from build123d import *

# Parameters (mm, degrees)
BOSS_EXTRUDE1_DEPTH = 0.75
SKETCH2_R           = 15.265
CUT_EXTRUDE1_DEPTH  = 47.8


with BuildPart() as part:
    # Sketch1 → Boss-Extrude1 (new body, symmetric)
    with BuildSketch(Plane.XY):
        Polygon((0, 15.245), (12, 41.045), (-34.1, 41.045), (-46.8, 15.245), align=None)
    extrude(amount=BOSS_EXTRUDE1_DEPTH, both=True)

    # Sketch2 → Cut-Extrude1 (cut, through all)
    with BuildSketch(Plane(origin=(0, 0, 0), x_dir=(0, 0, -1), z_dir=(1, 0, 0))):
        Circle(SKETCH2_R)
    extrude(amount=-CUT_EXTRUDE1_DEPTH, mode=Mode.SUBTRACT)


solid = part.part
Could you check a few things on this model? Use its own coordinates, in mm. Coordinates: 2 decimals unless noted, no trailing zeros. Loops run counter-clockwise (first coordinate to the right, second up) from the corner with the lowest first, then second, coordinate; pieces in that order, holes last.
1. Imagine slicing it at A-A (z = 0.1). Please give me the cut outline in (x, y) (3 decimals).
2. I need wall thicknesses on L1, parallel to Y at x = -25, z = -0.35 (3 decimals); L2, parallel to X at y = 26.75, z = 0.25; L3, parallel to X at y = 32.5, z = 0.1. Which ranges of each line are inside material? Lowest first, please.
3. Imagine slicing it at B-B (y = 18.75). Please give me the cut outline in (x, z), and give its area (3 significant figures).
4. Imagine slicing it at C-C (y = 38). Please give me the cut outline in (x, z).
Computed values:
1. outline: (-46.79, 15.265) - (0, 15.265) - (0, 15.245) - (12, 41.045) - (-34.1, 41.045) - close
2. L1: y = 15.261 to 41.045
2. L2: x = -41.14 to 5.35
2. L3: x = -38.31 to 8.03
3. outline: (-45.07, -0.75) - (1.63, -0.75) - (1.63, 0.75) - (-45.07, 0.75) - close
3. area: 70.1 mm2
4. outline: (-35.6, -0.75) - (10.58, -0.75) - (10.58, 0.75) - (-35.6, 0.75) - close
